Geometry check sheet. Reference: drawing and pictorial views, mm from the part's lowest x, y, z. A direction names the side the tool comes from. Give positions to 0.01 mm unless a question says otherwise; leave off trailing zeros. Loops run counter-clockwise (first coordinate to the right, second up) from the corner with the lowest first, then second, coordinate; pieces in that order, holes last. Notation, with made-up numbers: (79.5, 43.5) -> (101.5, 43.5) arc R9 cw to (101.5, 54.5) -> close; hole circle Ø9 at (23.25, -9). An arc over 180 degrees is marked (long way). One line per item, written item: value. Start each with the question number.
(1) Gauge pin test, flat ends, axial feed: pin 1 Ø2 at (x, z) = (13, 12.5) entering from +Y; pin 2 Ø2.5 at (x, y) = (40.5, 14.35) entering from +Z; pin 3 Ø4 at (x, y) = (9.5, 45.35) entering from +Z. Record the tip position at first contact, or that the pin passes through.
(2) Sectioned sample at A-A, the plane x = 25. Record the cut outline in (y, z), then the cut area to 4 significant figures.
(3) Sectioned sample at C-C, the plane z = 32.5. Record the cut outline in (x, y), then the cut area to 3 significant figures.
(4) Sectioned sample at B-B, the plane y = 45.35. Record the cut outline in (x, z), then the cut area to 3 significant figures.
(5) Scan lines: line 1 along Y through (x, z) = (40.5, 1.8); line 2 along X through (y, z) = (14, 2); line 3 along Y through (x, z) = (9.5, 0.9). Record each from-to range of solid material in increasing order. Write a range as from..to.
(6) Tool access check on the marked faces 1 and 2. Record the directions out of +Z, -Z, +X, -X, +Y, -Y that give a thin tool (end or side, any length) a straight path to the whole face; none if there is none.
(7) Sectioned sample at D-D, the plane y = 29.85. Record the cut outline in (x, z).
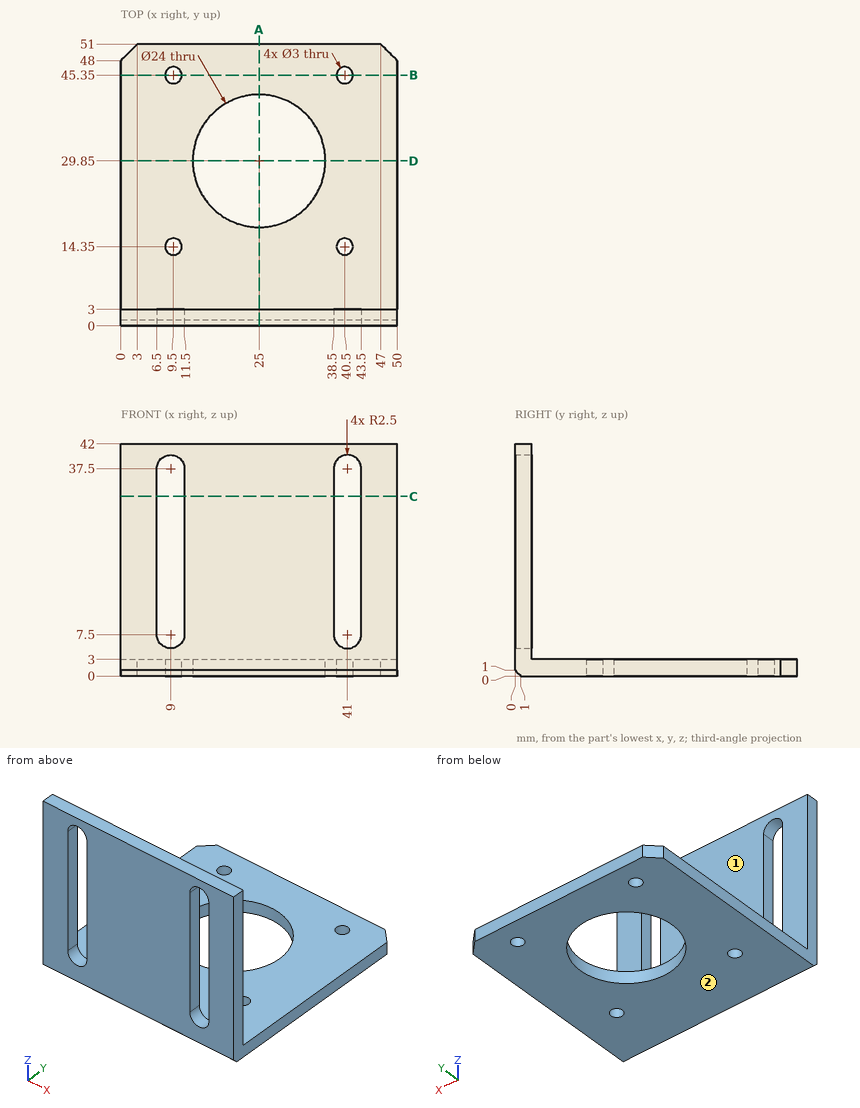
Calculated:
1. pin 1: stops at y = 3
1. pin 2: passes through
1. pin 3: stops at z = 3
2. outline: (0, 1) -> (1, 0) -> (17.85, 0) -> (17.85, 3) -> (3, 3) -> (3, 42) -> (0, 42) -> close; (41.85, 0) -> (51, 0) -> (51, 3) -> (41.85, 3) -> close
2. area: 197.5 mm2
3. outline: (0, 0) -> (6.5, 0) -> (6.5, 3) -> (0, 3) -> close; (11.5, 0) -> (38.5, 0) -> (38.5, 3) -> (11.5, 3) -> close; (43.5, 0) -> (50, 0) -> (50, 3) -> (43.5, 3) -> close
3. area: 120 mm2
4. outline: (0, 0) -> (8, 0) -> (8, 3) -> (0, 3) -> close; (11, 0) -> (39, 0) -> (39, 3) -> (11, 3) -> close; (42, 0) -> (50, 0) -> (50, 3) -> (42, 3) -> close
4. area: 132 mm2
5. line 1: y = 0..12.85, 15.85..43.85, 46.85..51
5. line 2: x = 0..8.04, 10.96..39.04, 41.96..50
5. line 3: y = 0.1..12.85, 15.85..43.85, 46.85..51
6. face 1: +Z, +X, -X, +Y
6. face 2: -Z, +X, -X, +Y, -Y
7. outline: (0, 0) -> (13, 0) -> (13, 3) -> (0, 3) -> close; (37, 0) -> (50, 0) -> (50, 3) -> (37, 3) -> close
